Geometry check sheet. Reference: drawing and pictorial views, mm from the part's lowest x, y, z. A direction names the side the tool comes from. Round coordinates to 2 decimals unless told otherwise and drop trailing zeros. Order: outer loops, then holes, each group sorted by start corner. A loop starts at its lowest first (then second) coordinate and runs counter-clockwise, first axis right, second up.
(1) Cross-section at B-B on x = 31.25. Enter the section's corners in (y, z).
(2) Cross-section at D-D on z = 4. Enter the section's corners in (x, y).
(3) Cross-section at C-C on y = 1.45. Count the separate pieces of the cut face and the enclosed holes in it, and give its area (3 significant figures).
(4) Gauge pin test, flat ends, axial feed: P1, Ø0.9, axis at y = 3.5, z = 18, coming from the -X side; P2, Ø4, axis at x = 3.75, z = 10.4, coming from the +Y side; P3, Ø2.5, axis at x = 31.25, z = 10.4, coming from the +Y side; P4, Ø1.5, axis at y = 4, z = 19, coming from the +X side. Record the tip position at first contact, or that the pin passes through.
(5) Thickness scan on L1, parallel to X at y = 1.45, z = 30.4; L2, parallel to X at y = 0.65, z = 31; L3, parallel to Z at x = 4, y = 1.15. Record the ranges inside material, lowest first.
(6) Cross-section at A-A on z = 20.4. Enter the section's corners in (x, y), and give its area (3 significant figures).
(7) Set-up check for the marked faces 1, 2 and 3: record each of +Z, -Z, +X, -X, +Y, -Y from which the full face is reachable in a straight line by a thin tool's end or side.
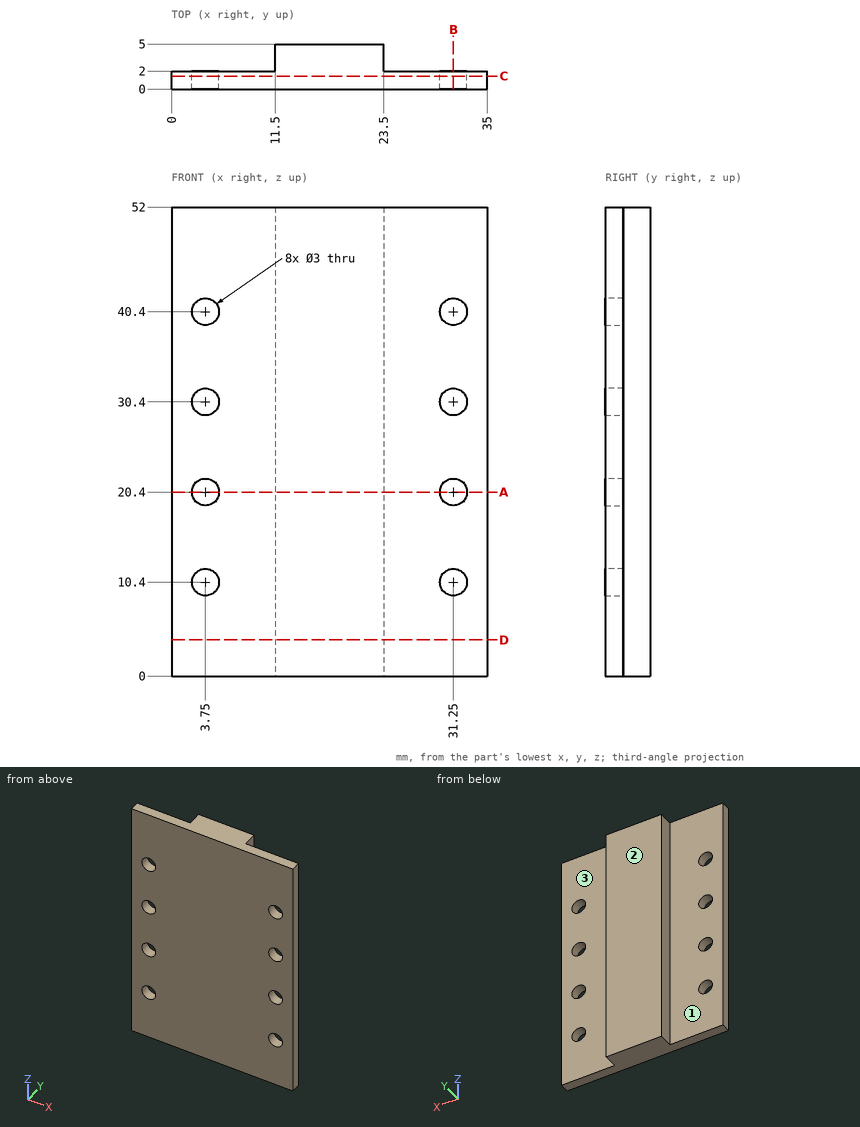
Found:
1. outline: (0, 0) - (2, 0) - (2, 8.9) - (0, 8.9) - close; (0, 11.9) - (2, 11.9) - (2, 18.9) - (0, 18.9) - close; (0, 21.9) - (2, 21.9) - (2, 28.9) - (0, 28.9) - close; (0, 31.9) - (2, 31.9) - (2, 38.9) - (0, 38.9) - close; (0, 41.9) - (2, 41.9) - (2, 52) - (0, 52) - close
2. outline: (0, 0) - (35, 0) - (35, 2) - (23.5, 2) - (23.5, 5) - (11.5, 5) - (11.5, 2) - (0, 2) - close
3. separate pieces: 1
3. enclosed holes: 8
3. area: 1,760 mm2
4. P1: stops at x = 11.5
4. P2: stops at y = 2
4. P3: passes through
4. P4: stops at x = 23.5
5. L1: x = 0 to 2.25, 5.25 to 29.75, 32.75 to 35
5. L2: x = 0 to 2.38, 5.12 to 29.88, 32.62 to 35
5. L3: z = 0 to 8.92, 11.88 to 18.92, 21.88 to 28.92, 31.88 to 38.92, 41.88 to 52
6. outline: (0, 0) - (2.25, 0) - (2.25, 2) - (0, 2) - close; (5.25, 0) - (29.75, 0) - (29.75, 2) - (23.5, 2) - (23.5, 5) - (11.5, 5) - (11.5, 2) - (5.25, 2) - close; (32.75, 0) - (35, 0) - (35, 2) - (32.75, 2) - close
6. area: 94.0 mm2
7. face 1: +Z, -Z, -X, +Y
7. face 2: +Z, -Z, +X, -X, +Y
7. face 3: +Z, -Z, +X, +Y
